Design review of the part built by this model. Coordinates are the model's own, in mm. Coordinates: 2 decimals unless noted, no trailing zeros. Loops run counter-clockwise (first coordinate to the right, second up) from the corner with the lowest first, then second, coordinate; pieces in that order, holes last. Notation, with made-up numbers: (24.5, 37.25) -> (65.5, 37.25) arc R26 ccw to (65.5, 58.25) -> close; hole circle Ø11 at (84.25, 13.5). An arc over 180 degrees is marked (long way). Answer as a JSON object with one key per item and string values.
```python
from build123d import *

# Parameters (mm, degrees)
ESQUISSE1_R             = 3
BOSS_EXTRU_1_DEPTH      = 130
CONG_1_R                = 2
ESQUISSE2_W             = 6
ESQUISSE2_H             = 1.2
ENL_V_MAT_EXTRU_1_DEPTH = 131.069212347


with BuildPart() as part:
    # Esquisse1 → Boss.-Extru.1 (new body)
    with BuildSketch(Plane.XY):
        Circle(ESQUISSE1_R)
    extrude(amount=BOSS_EXTRU_1_DEPTH)

    # Congé1
    cong_1_edges = [part.edges().sort_by_distance(p)[0] for p in [
        (-3, 0, 0),
        (-3, 0, 130),
    ]]
    fillet(cong_1_edges, radius=CONG_1_R)

    # Esquisse2 → Enlèv. mat.-Extru.1 (cut, through all)
    with BuildSketch(Plane.XY.offset(130)):
        with Locations((0, 2.4)):
            Rectangle(ESQUISSE2_W, ESQUISSE2_H)
    extrude(amount=-ENL_V_MAT_EXTRU_1_DEPTH, mode=Mode.SUBTRACT)


solid = part.part
```
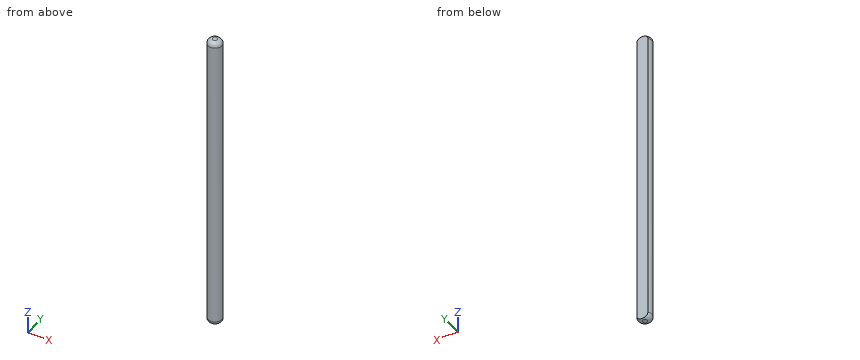
1) Wall thickness on probe 1 along X at (y, z) = (0.2, 62); probe 2 along Y at (x, z) = (-0.25, 11.5); probe 3 along Z at (x, y) = (-1.5, 0.9): over which ranges is each line inside the solid? List them lowest first.
Completed:
{"probe 1": "-2.99 to 2.99", "probe 2": "-2.99 to 1.8", "probe 3": "0.15 to 129.85"}
2) Clearance check with a flat-ended pin moving along its axis: pin 1 Ø1.5 at (y, z) = (-1, 78) entering from +X. State where the tip first meets the part, or that it passes through.
Completed:
{"pin 1": "x = 2.99"}
3) Add section A-A, the plane z = 27. Give the boundary of the cut face in (x, y).
Completed:
{"outline": "(-2.4, 1.8) arc R3 ccw (long way) to (2.4, 1.8) -> close"}
